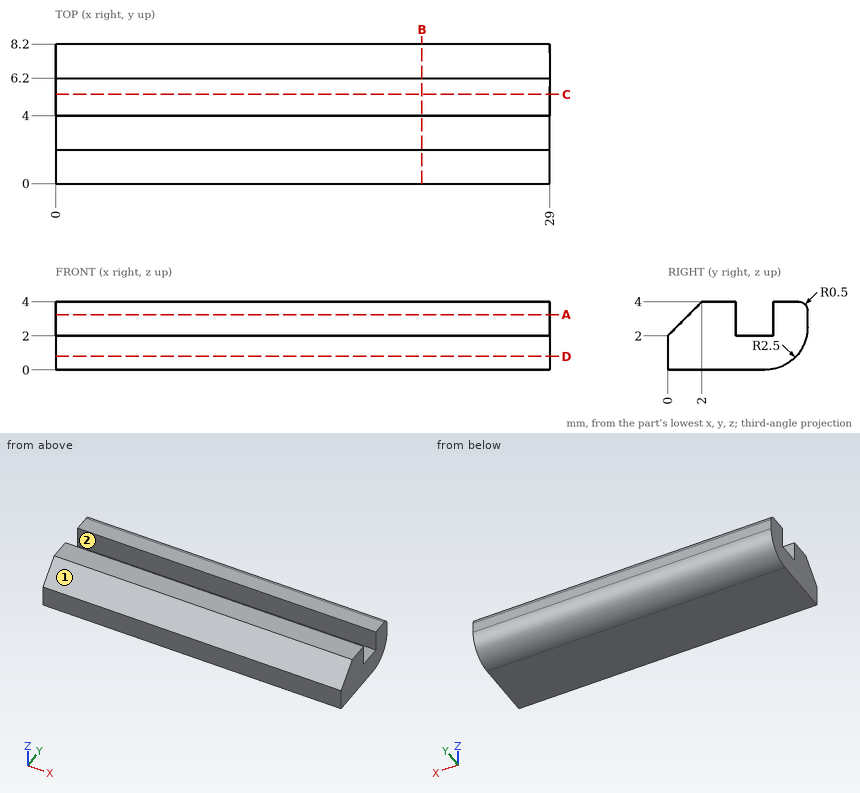
Could you check a few things on this drawing? It's one solid part, dimensions in mm from its lowest x, y, z. A direction names the side the tool comes from. Give positions to 0.01 mm unless a question says otherwise; leave off trailing zeros. Loops run counter-clockwise (first coordinate to the right, second up) from the corner with the lowest first, then second, coordinate; pieces in that order, holes last. Notation, with made-up numbers: M -22.75,51.5 L 16.25,51.5 A27 cw 16.25,83.5 Z; hole C 89.25,-7 d5. An arc over 180 degrees is marked long. Answer as a JSON object with one key per item and string values.
Q1. Suppose I cut it at B-B, the plane x = 21.5. List the corners of the cut face in (y, z) for me.
Values found:
{"outline": "M 0,0 L 5.7,0 A2.5 ccw 8.2,2.5 L 8.2,3.5 A0.5 ccw 7.7,4 L 6.2,4 L 6.2,2 L 4,2 L 4,4 L 2,4 L 0,2 Z"}
Q2. Suppose I cut it at A-A, the plane z = 3.25. List the corners of the cut face in (x, y) for me.
Values found:
{"outline": "M 0,1.25 L 29,1.25 L 29,4 L 0,4 Z; M 0,6.2 L 29,6.2 L 29,8.2 L 0,8.2 Z"}
Q3. For P1, Ø0.7, axis at x = 12, y = 5, coming from the +Z side, with a flat end and sliding along its axis, tell me the tip position at first contact or that it passes through.
Values found:
{"P1": "stops at z = 2"}
Q4. If I drill on probe 1 along Z at (x, y) = (3, 1.5); probe 2 along Z at (x, y) = (5, 5.75); probe 3 along Y at (x, z) = (16.5, 2.95), over which ranges is the centre line in solid material (lowest first)? Write a range as [from, to].
Values found:
{"probe 1": "z = [0, 3.5]", "probe 2": "z = [0, 2]", "probe 3": "y = [0.95, 4], [6.2, 8.2]"}
Q5. Suppose I cut it at C-C, the plane y = 5.25. List the corners of the cut face in (x, z) for me.
Values found:
{"outline": "M 0,0 L 29,0 L 29,2 L 0,2 Z"}
Q6. Suppose I cut it at D-D, the plane z = 0.8. List the corners of the cut face in (x, y) for me, plus the area to 3 significant figures.
Values found:
{"outline": "M 0,0 L 29,0 L 29,7.53 L 0,7.53 Z", "area": "218 mm²"}
Q7. For the marked faces 1 and 2, which set-ups out of +Z, -Z, +X, -X, +Y, -Y let a thin tool reach every point of the face, with its end or its side?
Values found:
{"face 1": "+Z, +X, -X, -Y", "face 2": "+Z, +X, -X"}
